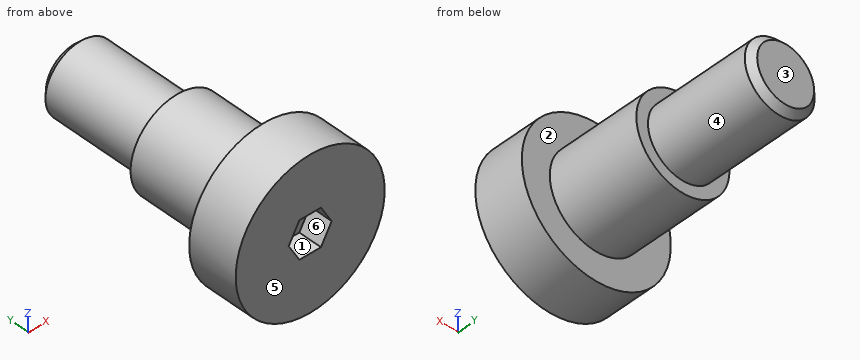
```python
from build123d import *

# Parameters (mm, degrees)
SKETCH_1_R          = 6.4
EXTRUDE_1_DEPTH     = 4.3
SKETCH_2_R          = 4
EXTRUDE_2_DEPTH     = 8
SKETCH_3_R          = 3
EXTRUDE_3_DEPTH     = 9.5
CUT_EXTRUDE_1_DEPTH = 2


# Read off the part's stored shape, not the designer's step: M6x1.0 机械螺纹 螺柱1
with BuildPart() as part:
    # 草图1 → 凸台-拉伸1 (new body)
    with BuildSketch(Plane(origin=(0, 0, 0), x_dir=(1, 0, 0), z_dir=(0, 1, 0))):
        with Locations(Location((0, 0, 0), (0, 0, 90))):
            Circle(SKETCH_1_R)
    extrude(amount=EXTRUDE_1_DEPTH)

    # 草图2 → 凸台-拉伸2 (add)
    with BuildSketch(Plane(origin=(0, 4.3, 0), x_dir=(1, 0, 0), z_dir=(0, 1, 0))):
        with Locations(Location((0, 0, 0), (0, 0, 270))):
            Circle(SKETCH_2_R)
    extrude(amount=EXTRUDE_2_DEPTH)

    # 草图3 → 凸台-拉伸3 (add)
    with BuildSketch(Plane(origin=(0, 12.3, 0), x_dir=(1, 0, 0), z_dir=(0, 1, 0))):
        with Locations(Location((0, 0, 0), (0, 0, 270))):
            Circle(SKETCH_3_R)
    extrude(amount=EXTRUDE_3_DEPTH)

    # M6x1.0 机械螺纹 螺柱1 outline → M6x1.0 机械螺纹 螺柱1 (revolve, cut)
    with BuildSketch(Plane.XY):
        Polygon((3, 21.8), (2.4455, 21.8), (3, 21.2455), align=None)
    revolve(axis=Axis((0, 0, 0), (0, 1, 0)), mode=Mode.SUBTRACT)

    # 草图5 → 切除-拉伸1 (cut)
    with BuildSketch(Plane.XZ):
        Polygon((1.847520861, 0), (0.923760431, 1.6), (-0.923760431, 1.6), (-1.847520861, 0), (-0.923760431, -1.6), (0.923760431, -1.6), align=None)
    extrude(amount=-CUT_EXTRUDE_1_DEPTH, mode=Mode.SUBTRACT)


solid = part.part
```
Source: CAD feature listing. Evaluate the final solid. Frame: model axes, mm. Face numbers are marked on the shaded views. A direction names the side the tool comes from. Give positions to 0.01 mm unless a question says otherwise; leave off trailing zeros. Write each loop counter-clockwise with the first axis right and the second up, starting at its lowest first coordinate (ties: lowest second). Pieces come first, ordered by that corner, then holes.
1. First-contact query: pin 1 (5 mm diameter, centred on x = -2.5, y = 10.5, fed in from +Z); pin 2 (4 mm diameter, centred on x = -4, y = 8.5, fed in from +Z); pin 3 (3 mm diameter, centred on y = 10, z = -3.5, fed in from +X). Flat tips, straight axial feed; report the tip coordinate or a pass-through.
2. Access query for the marked faces 1, 2 and 3. Directions: +Z, -Z, +X, -X, +Y, -Y. A direction counts if a zero-diameter tool reaches every point of the face in a straight line with its end or side. Return the directions, or none.
3. Section query A-A (x = 0). Return the cut outline in (y, z), then the cut area to 3 significant figures.
4. Section query C-C (z = -3.25). Return the cut outline in (x, y).
5. Section query B-B (y = 9.5). Return the cut outline in (x, z), then the cut area to 3 significant figures.
6. Material intervals for line 1 along Y through (x, z) = (5.75, 1); line 2 along Y through (x, z) = (-0.75, -1); line 3 along X through (y, z) = (17, 1), sorted ascending.
7. Section query D-D (x = -3.5). Return the cut outline in (y, z), then the cut area to 3 significant figures.
8. Pull-direction query (X, two-part tool) for the marked faces 4, 5 and 6; classes: +X half, -X half, draft (parallel to the pull), parting line (faces both ways), or undercut.
Output values:
1. pin 1: stops at z = 4
1. pin 2: stops at z = 3.46
1. pin 3: stops at x = 3.46
2. face 1: -Y
2. face 2: +Y
2. face 3: +Z, -Z, +X, -X, +Y
3. outline: (0, -6.4) - (4.3, -6.4) - (4.3, -4) - (12.3, -4) - (12.3, -3) - (21.25, -3) - (21.8, -2.45) - (21.8, 2.45) - (21.25, 3) - (12.3, 3) - (12.3, 4) - (4.3, 4) - (4.3, 6.4) - (0, 6.4) - (0, 1.6) - (2, 1.6) - (2, -1.6) - (0, -1.6) - close
3. area: 169 mm2
4. outline: (-5.51, 0) - (5.51, 0) - (5.51, 4.3) - (2.33, 4.3) - (2.33, 12.3) - (-2.33, 12.3) - (-2.33, 4.3) - (-5.51, 4.3) - close
5. outline: circle Ø8 at (0, 0)
5. area: 50.3 mm2
6. line 1: y = 0 to 4.3
6. line 2: y = 2 to 21.8
6. line 3: x = -2.83 to 2.83
7. outline: (0, -5.36) - (4.3, -5.36) - (4.3, -1.94) - (12.3, -1.94) - (12.3, 1.94) - (4.3, 1.94) - (4.3, 5.36) - (0, 5.36) - close
7. area: 77.1 mm2
8. face 4: parting line
8. face 5: draft
8. face 6: undercut
